Can you work these out from the model? Positions are in its coordinate system, mm. A direction names the side the tool comes from. Give positions to 0.01 mm unless a question says otherwise; leave off trailing zeros. Write each loop counter-clockwise with the first axis right and the second up, starting at its lowest first coordinate (ties: lowest second). Pieces come first, ordered by that corner, then holes. Notation, with made-up numbers: (41.5, 23) - (69.5, 23) arc R21 ccw to (69.5, 48) - close; hole circle Ø4 at (52, -36.75). An arc over 180 degrees is marked (long way). Return JSON: item names as keys, results as strings. Group by question number.
from build123d import *

# Parameters (mm, degrees)
SKETCH1_W           = 115
SKETCH1_H           = 45
SKETCH1_R           = 4
SKETCH1_R_2         = 1.5
BOSS_EXTRUDE1_DEPTH = 8
SKETCH2_W           = 8
SKETCH2_H           = 10
SKETCH2_H_2         = 8
CUT_EXTRUDE1_DEPTH  = 16
FILLET1_R           = 3
SKETCH4_R           = 1.5
CUT_EXTRUDE2_DEPTH  = 16


with BuildPart() as part:
    # Sketch1 → Boss-Extrude1 (new body)
    with BuildSketch(Plane(origin=(0, 0, 0), x_dir=(1, 0, 0), z_dir=(0, 1, 0))):
        Rectangle(SKETCH1_W, SKETCH1_H)
        with Locations(Location((0, 0, 0), (0, 0, 270))):
            Circle(SKETCH1_R, mode=Mode.SUBTRACT)
        with Locations(Location((0, 13, 0), (0, 0, 270))):
            Circle(SKETCH1_R_2, mode=Mode.SUBTRACT)
        with Locations(Location((11.258330249, -6.5, 0), (0, 0, 270))):
            Circle(SKETCH1_R_2, mode=Mode.SUBTRACT)
        with Locations(Location((-11.258330249, -6.5, 0), (0, 0, 270))):
            Circle(SKETCH1_R_2, mode=Mode.SUBTRACT)
    extrude(amount=BOSS_EXTRUDE1_DEPTH)

    # Sketch2 → Cut-Extrude1 (cut)
    with BuildSketch(Plane(origin=(0, 8, 0), x_dir=(1, 0, 0), z_dir=(0, 1, 0))):
        with Locations((-39, 0)):
            Rectangle(SKETCH2_W, SKETCH2_H)
        with Locations((-39, 18.82979477)):
            Rectangle(SKETCH2_W, SKETCH2_H_2)
        with Locations((39, 18.82979477)):
            Rectangle(SKETCH2_W, SKETCH2_H_2)
        with Locations((39, 0)):
            Rectangle(SKETCH2_W, SKETCH2_H)
        with Locations((-39, -18.5)):
            Rectangle(SKETCH2_W, SKETCH2_H_2)
        with Locations((39, -18.5)):
            Rectangle(SKETCH2_W, SKETCH2_H_2)
    extrude(amount=-CUT_EXTRUDE1_DEPTH, mode=Mode.SUBTRACT)

    # Fillet1
    fillet1_edges = [part.edges().sort_by_distance(p)[0] for p in [
        (-57.5, 4, 22.5),
        (-57.5, 4, -22.5),
        (57.5, 4, -22.5),
        (57.5, 4, 22.5),
    ]]
    fillet(fillet1_edges, radius=FILLET1_R)

    # Sketch4 → Cut-Extrude2 (cut)
    with BuildSketch(Plane(origin=(0, 8, 0), x_dir=(1, 0, 0), z_dir=(0, 1, 0))):
        with Locations(Location((52.5, 14.5, 0), (0, 0, 270))):
            Circle(SKETCH4_R)
        with Locations(Location((-52.5, 14.5, 0), (0, 0, 270))):
            Circle(SKETCH4_R)
        with Locations(Location((-52.5, -14.5, 0), (0, 0, 270))):
            Circle(SKETCH4_R)
        with Locations(Location((52.5, -14.5, 0), (0, 0, 270))):
            Circle(SKETCH4_R)
    extrude(amount=-CUT_EXTRUDE2_DEPTH, mode=Mode.SUBTRACT)


solid = part.part
1) Imagine slicing it at B-B, the plane z = 6.5. Write out the boundary of the cut face in (x, y).
2) Imagine slicing it at C-C, the plane z = -1.5. Write out the boundary of the cut face in (x, y).
3) On a 3-axis mill with a long thin cutter (end or side, diameter ignored), from which of +Z, -Z, +X, -X, +Y, -Y can I reach the whole of each face in a straight line? I mean faces 5 (the face through (43, 4, 0)), 6 (the face through (-35, 4, -19)), 7 (the face through (35, 4, 19)). Say none if no direction works.
4) Imagine slicing it at A-A, the plane x = -52.5. Write out the boundary of the cut face in (y, z).
5) I need wall thicknesses on line 1 along X through (y, z) = (4.5, 6.5); line 2 along X through (y, z) = (7.25, -16.5); line 3 along X through (y, z) = (1.5, -14). Which ranges of each line are inside material? Lowest first, please.
6) Will these pins go through, and if not, where does the flat tip stop? pin 1 Ø4 at (x, y) = (38.5, 5) entering from -Z; pin 2 Ø2.5 at (x, y) = (37.5, 4) entering from +Z.
7) We'd pull the mould along Z, two halves only. Please class faces 1 (the face through (56.6, 4.06, -21.64)), 2 (the face through (35, 4, -19)), 3 (the face through (51.036, 4.056, 14.175)), 4 (the face through (-39, 4, 14.5)): pulls with the +Z half, pulls with the -Z half, needs draft (parallel to the pull), parting line crosses it, or undercut.
8) Imagine slicing it at D-D, the plane y = 3. Count the separate pieces of the cut face and the enclosed holes in it, and give its area (3 significant figures).
Resolved:
{
 "1": {"outline": "(-57.5, 0) - (-12.76, 0) - (-12.76, 8) - (-57.5, 8) - close; (-9.76, 0) - (9.76, 0) - (9.76, 8) - (-9.76, 8) - close; (12.76, 0) - (57.5, 0) - (57.5, 8) - (12.76, 8) - close"},
 "2": {"outline": "(-57.5, 0) - (-43, 0) - (-43, 8) - (-57.5, 8) - close; (-35, 0) - (-3.71, 0) - (-3.71, 8) - (-35, 8) - close; (3.71, 0) - (35, 0) - (35, 8) - (3.71, 8) - close; (43, 0) - (57.5, 0) - (57.5, 8) - (43, 8) - close"},
 "3": {"face 5": "+Y, -Y", "face 6": "-Z, +Y, -Y", "face 7": "+Z, +Y, -Y"},
 "4": {"outline": "(0, -22.5) - (8, -22.5) - (8, -16) - (0, -16) - close; (0, -13) - (8, -13) - (8, 13) - (0, 13) - close; (0, 16) - (8, 16) - (8, 22.5) - (0, 22.5) - close"},
 "5": {"line 1": "-57.5 to -12.76, -9.76 to 9.76, 12.76 to 57.5", "line 2": "-57.5 to -43, -35 to 35, 43 to 57.5", "line 3": "-57.5 to -53.91, -51.09 to -1.12, 1.12 to 51.09, 53.91 to 57.5"},
 "6": {"pin 1": "z = -14.83", "pin 2": "z = 14.5"},
 "7": {"face 1": "pulls with the -Z half", "face 2": "needs draft", "face 3": "undercut", "face 4": "pulls with the +Z half"},
 "8": {"separate pieces": "1", "enclosed holes": "10", "area": "4,660 mm^2"}
}
